```python
from build123d import *

# Parameters (mm, degrees)
FILLET1_R = 0.5


with BuildPart() as part:
    # Sketch1 → Revolve1 (revolve)
    with BuildSketch(Plane.XZ):
        Polygon((6, -3.5), (6, -2.5), (9, -2.5), (9, -3.5), (11, -3.5), (11, 3.5), (9, 3.5), (9, 2.5), (6, 2.5), (6, 3.5), (4, 3.5), (4, -3.5), align=None)
    revolve(axis=Axis((0, 0, 3.5), (0, 0, -1)))

    # Fillet1
    fillet1_edges = [part.edges().sort_by_distance(p)[0] for p in [
        (-11, 0, 3.5),
        (-11, 0, -3.5),
    ]]
    fillet(fillet1_edges, radius=FILLET1_R)


solid = part.part
```
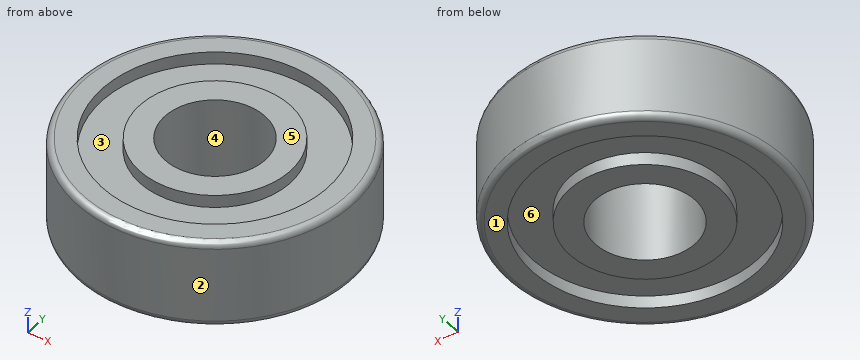
CAD build for the part. Positions are in the model's coordinates, mm. Face numbers are marked on the shaded views. A direction names the side the tool comes from. Give positions to 0.01 mm unless a question says otherwise; leave off trailing zeros. Loops run counter-clockwise (first coordinate to the right, second up) from the corner with the lowest first, then second, coordinate; pieces in that order, holes last. Notation, with made-up numbers: (32.25, 42) -> (81.25, 42) arc R21 ccw to (81.25, 78) -> close; hole circle Ø4 at (-28, 15). An arc over 180 degrees is marked (long way). Use a Markdown table: item, result.
1. Wall check: L1, parallel to X at y = 0, z = -2.8; L2, parallel to Y at x = 0, z = 1.25. Give the ranges that are in metal, low to high. Write a range as [from, to].
Check result:
| item | result |
|---|---|
| L1 | x = [-11, -9], [-6, -4], [4, 6], [9, 11] |
| L2 | y = [-11, -4], [4, 11] |
2. Which spindle directions (+Z, -Z, +X, -X, +Y, -Y) get a long thin tool onto all of the face, cutting with end or side? Do the marked faces 5 and 6. Say none if no direction does.
Check result:
| item | result |
|---|---|
| face 5 | +Z, +X, -X, +Y, -Y |
| face 6 | -Z |
3. Slice it at C-C (z = -1). List the corners of the cut face in (x, y), plus the area to 3 significant figures.
Check result:
| item | result |
|---|---|
| outline | circle Ø22 at (0, 0); hole circle Ø8 at (0, 0) |
| area | 330 mm^2 |
4. Mould opens along Y. For the marked faces 1, 2, 3 and 4 say: pulls with the +Y half, pulls with the -Y half, needs draft (parallel to the pull), parting line crosses it, or undercut.
Check result:
| item | result |
|---|---|
| face 1 | needs draft |
| face 2 | parting line crosses it |
| face 3 | undercut |
| face 4 | undercut |
5. Slice it at A-A (x = 0). List the corners of the cut face in (y, z), plus the area to 3 significant figures.
Check result:
| item | result |
|---|---|
| outline | (-11, -3) arc R0.5 ccw to (-10.5, -3.5) -> (-9, -3.5) -> (-9, -2.5) -> (-6, -2.5) -> (-6, -3.5) -> (-4, -3.5) -> (-4, 3.5) -> (-6, 3.5) -> (-6, 2.5) -> (-9, 2.5) -> (-9, 3.5) -> (-10.5, 3.5) arc R0.5 ccw to (-11, 3) -> close; (4, -3.5) -> (6, -3.5) -> (6, -2.5) -> (9, -2.5) -> (9, -3.5) -> (10.5, -3.5) arc R0.5 ccw to (11, -3) -> (11, 3) arc R0.5 ccw to (10.5, 3.5) -> (9, 3.5) -> (9, 2.5) -> (6, 2.5) -> (6, 3.5) -> (4, 3.5) -> close |
| area | 85.8 mm^2 |
6. Flat gauge pins, fed straight in: pin 1 (6.5 mm diameter, centred on x = 0, y = 0, fed in from -Z); pin 2 (1.5 mm diameter, centred on y = -2, z = 1.5, fed in from -X); pin 3 (3 mm diameter, centred on x = -0.5, z = 1.5, fed in from -Y); pin 4 (2 mm diameter, centred on x = -2.5, z = 2, fed in from +Y). Where does each tip first touch, or does it go through?
Check result:
| item | result |
|---|---|
| pin 1 | passes through |
| pin 2 | stops at x = -10.93 |
| pin 3 | stops at y = -11 |
| pin 4 | stops at y = 10.9 |
